Verification items for the finished model (mm, model axes). Face numbers are marked on the shaded views. Give positions to 0.01 mm unless a question says otherwise; leave off trailing zeros. Loops run counter-clockwise (first coordinate to the right, second up) from the corner with the lowest first, then second, coordinate; pieces in that order, holes last. Notation, with made-up numbers: (44, 16.25) - (49, 16.25) arc R10 ccw to (49, 25.25) - close; hole circle Ø3 at (-0.5, 36.5). An arc over 180 degrees is marked (long way). Answer in a Markdown table with one row per item.
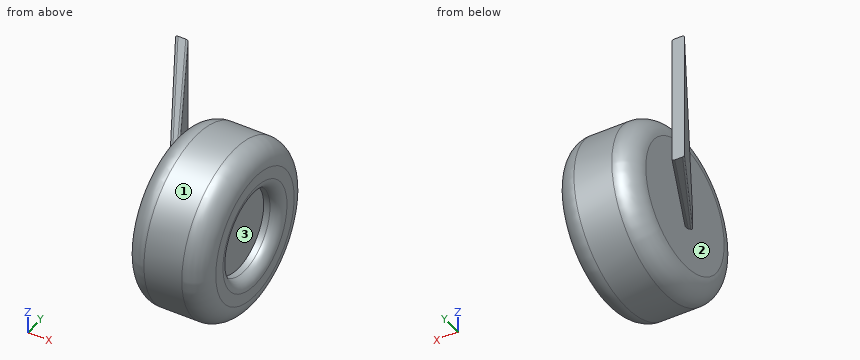
```python
from build123d import *

# Parameters (mm, degrees)
SKETCH1_R           = 201.5
SKETCH1_R_2         = 98.768091278
BOSS_EXTRUDE1_DEPTH = 190
SKETCH2_R           = 98.768091278
BOSS_EXTRUDE2_DEPTH = 150
FILLET1_R           = 50
FILLET2_R           = 25
BOSS_EXTRUDE3_DEPTH = 310
CUT_EXTRUDE5_DEPTH  = 300
FILLET3_R           = 5


with BuildPart() as part:
    # Sketch1 → Boss-Extrude1 (new body)
    with BuildSketch(Plane(origin=(0, 0, 0), x_dir=(0, 0, -1), z_dir=(1, 0, 0))):
        Circle(SKETCH1_R)
        Circle(SKETCH1_R_2, mode=Mode.SUBTRACT)
    extrude(amount=BOSS_EXTRUDE1_DEPTH)

    # Sketch2 → Boss-Extrude2 (add)
    with BuildSketch(Plane.ZY):
        Circle(SKETCH2_R)
    extrude(amount=-BOSS_EXTRUDE2_DEPTH)

    # Fillet1
    fillet1_edges = [part.edges().sort_by_distance(p)[0] for p in [
        (0, 0, 201.5),
        (190, 0, 201.5),
    ]]
    fillet(fillet1_edges, radius=FILLET1_R)

    # Fillet2
    fillet2_edges = [part.edges().sort_by_distance(p)[0] for p in [
        (190, 0, 98.768091278),
    ]]
    fillet(fillet2_edges, radius=FILLET2_R)

    # Sketch4 → Boss-Extrude3 (add)
    with BuildSketch(Plane.XY):
        Polygon((0, 0), (-265, 481.949167444), (-295, 481.949167444), (0, -30), align=None)
    extrude(amount=-BOSS_EXTRUDE3_DEPTH)

    # Sketch5 → Cut-Extrude5 (cut)
    with BuildSketch(Plane.ZY.offset(300)):
        Polygon((-310, 481.949167444), (-40, -30), (-310, -30), align=None)
    extrude(amount=-CUT_EXTRUDE5_DEPTH, mode=Mode.SUBTRACT)

    # Fillet3
    fillet3_edges = [part.edges().sort_by_distance(p)[0] for p in [
        (-132.5, 240.974583722, 0),
        (-147.5, 225.974583722, 0),
        (-147.5, 225.974583722, -175),
        (-132.5, 240.974583722, -182.910941667),
    ]]
    fillet(fillet3_edges, radius=FILLET3_R)


solid = part.part
```
Q1. Go/stop test with flat-tipped pins: P1, Ø1, axis at x = -208, z = -93, coming from the -Y side; P2, Ø3, axis at y = 244, z = -72.5, coming from the -X side. Record where each tip stops, or that it passes through.
Completed:
| item | result |
|---|---|
| P1 | y = 330.1 |
| P2 | x = -158.75 |
Q2. Draft check along X on the marked faces 1, 2 and 3. Enter one of: +X half, -X half, draft (parallel to the pull), parting line (faces both ways), or undercut.
Completed:
| item | result |
|---|---|
| face 1 | draft |
| face 2 | undercut |
| face 3 | +X half |
Q3. Thickness scan on line 1 (Y direction, x = 155.25, z = 0); line 2 (Y direction, x = 158.75, z = 0); line 3 (X direction, y = 174, z = -1). Record the ranges inside material, lowest first.
Completed:
| item | result |
|---|---|
| line 1 | -199.12 to -98.77, 98.77 to 199.12 |
| line 2 | -197.85 to -98.77, 98.77 to 197.85 |
| line 3 | -115.24 to -97.96, 5.35 to 184.65 |
Q4. Sectioned sample at A-A (x = 27). Record the cut outline in (y, z), and give its area (3 significant figures).
Completed:
| item | result |
|---|---|
| outline | circle Ø391.79 at (0, 0) |
| area | 121,000 mm^2 |
